from build123d import *

# Parameters (mm, degrees)
BOSS_EXTRUDE1_DEPTH = 200
SKETCH4_R           = 20
SKETCH4_R_2         = 50
CUT_EXTRUDE1_DEPTH  = 313
SCALE1_SCALE        = 0.75


with BuildPart() as part:
    # Sketch1 → Boss-Extrude1 (new body)
    with BuildSketch(Plane(origin=(0, 0, 0), x_dir=(1, 0, 0), z_dir=(0, 1, 0))):
        Polygon((75, -250), (105, -250), (105, 250), (75, 250), (75, 50), (-75, 50), (-75, 250), (-105, 250), (-105, -250), (-75, -250), (-75, -50), (75, -50), align=None)
    extrude(amount=BOSS_EXTRUDE1_DEPTH)

    # Sketch4 → Cut-Extrude1 (cut)
    with BuildSketch(Plane.ZY.offset(105)):
        with Locations((125, 100)):
            Circle(SKETCH4_R)
        with Locations((-150, 100)):
            Circle(SKETCH4_R_2)
    extrude(amount=-CUT_EXTRUDE1_DEPTH, mode=Mode.SUBTRACT)


with BuildPart() as part_1:
    # Scale1: scaled about (0, 100, 7.246945107)
    add(part.part.scale(SCALE1_SCALE).moved(Location((0, 25, 1.811736277))))


solid = part_1.part
Geometry: final body of the model. Coordinates: model frame, mm. A direction names the side the tool comes from. Round coordinates to 2 decimals unless told otherwise and drop trailing zeros. Loops run counter-clockwise (first coordinate to the right, second up) from the corner with the lowest first, then second, coordinate; pieces in that order, holes last. Notation, with made-up numbers: M 43.25,-8 L 61.25,-8 A18 ccw 61.25,-4 Z; hole C 35,-26 d6. An arc over 180 degrees is marked long. Put each result on its own line as item: value. Start each with the question number.
(1) Section query A-A (z = 155). Return loops of the section in (x, y), then the cut area to 3 significant figures.
(2) Material intervals for line 1 along X through (y, z) = (150.5, 104.5); line 2 along Z through (x, y) = (-48.5, 57.5); line 3 along Z through (x, y) = (59.5, 82), sorted ascending. Write a range as [from, to].
(3) Contact query for a flat-ended pin moving along its axis: pin 1 Ø5 at (x, y) = (4, 123.5) entering from -Z. Output: stop coordinate, or through.
(4) Set-up query: faces 4 (the face through (-56.25, 99, 115)), 5 (the face through (-67.7, 131.6, -90.5)), 6 (the face through (1, 99, -35.688)). Return all of +Z, -Z, +X, -X, +Y, -Y with unobstructed straight access to the full face (end or side cutting, diameter ignored); none if empty.
(5) Draft query along Y for faces 1 (the face through (-56.25, 66, -93)), 2 (the face through (5, 25, 1)), 3 (the face through (67.3, 131.6, -90.5)). Return one class per face: +Y half, -Y half, draft (parallel to the pull), parting line (faces both ways), or undercut.
(6) Section query C-C (z = -115). Return loops of the section in (x, y).
(7) Section query B-B (y = 100). Return loops of the section in (x, z).
(8) Section query D-D (y = 39). Return loops of the section in (x, z).
Findings below:
1. outline: M -78.75,25 L -56.25,25 L -56.25,175 L -78.75,175 Z; M 56.25,25 L 78.75,25 L 78.75,175 L 56.25,175 Z
1. area: 6,750 mm2
2. line 1: x = [-78.75, -56.25], [56.25, 78.75]
2. line 2: z = [-35.69, 39.31]
2. line 3: z = [-185.69, -143.59], [-77.79, 189.31]
3. pin 1: stops at z = -35.69
4. face 4: +Z, +Y, -Y
4. face 5: +X, -X
4. face 6: -Z, +Y, -Y
5. face 1: draft
5. face 2: -Y half
5. face 3: undercut
6. outline: M -78.75,25 L -56.25,25 L -56.25,62.75 L -78.75,62.75 Z; M -78.75,137.25 L -56.25,137.25 L -56.25,175 L -78.75,175 Z; M 56.25,25 L 78.75,25 L 78.75,62.75 L 56.25,62.75 Z; M 56.25,137.25 L 78.75,137.25 L 78.75,175 L 56.25,175 Z
7. outline: M -78.75,-185.69 L -56.25,-185.69 L -56.25,-148.19 L -78.75,-148.19 Z; M -78.75,-73.19 L -56.25,-73.19 L -56.25,-35.69 L 56.25,-35.69 L 56.25,-73.19 L 78.75,-73.19 L 78.75,80.56 L 56.25,80.56 L 56.25,39.31 L -56.25,39.31 L -56.25,80.56 L -78.75,80.56 Z; M -78.75,110.56 L -56.25,110.56 L -56.25,189.31 L -78.75,189.31 Z; M 56.25,-185.69 L 78.75,-185.69 L 78.75,-148.19 L 56.25,-148.19 Z; M 56.25,110.56 L 78.75,110.56 L 78.75,189.31 L 56.25,189.31 Z
8. outline: M -78.75,-185.69 L -56.25,-185.69 L -56.25,-35.69 L 56.25,-35.69 L 56.25,-185.69 L 78.75,-185.69 L 78.75,189.31 L 56.25,189.31 L 56.25,39.31 L -56.25,39.31 L -56.25,189.31 L -78.75,189.31 Z
